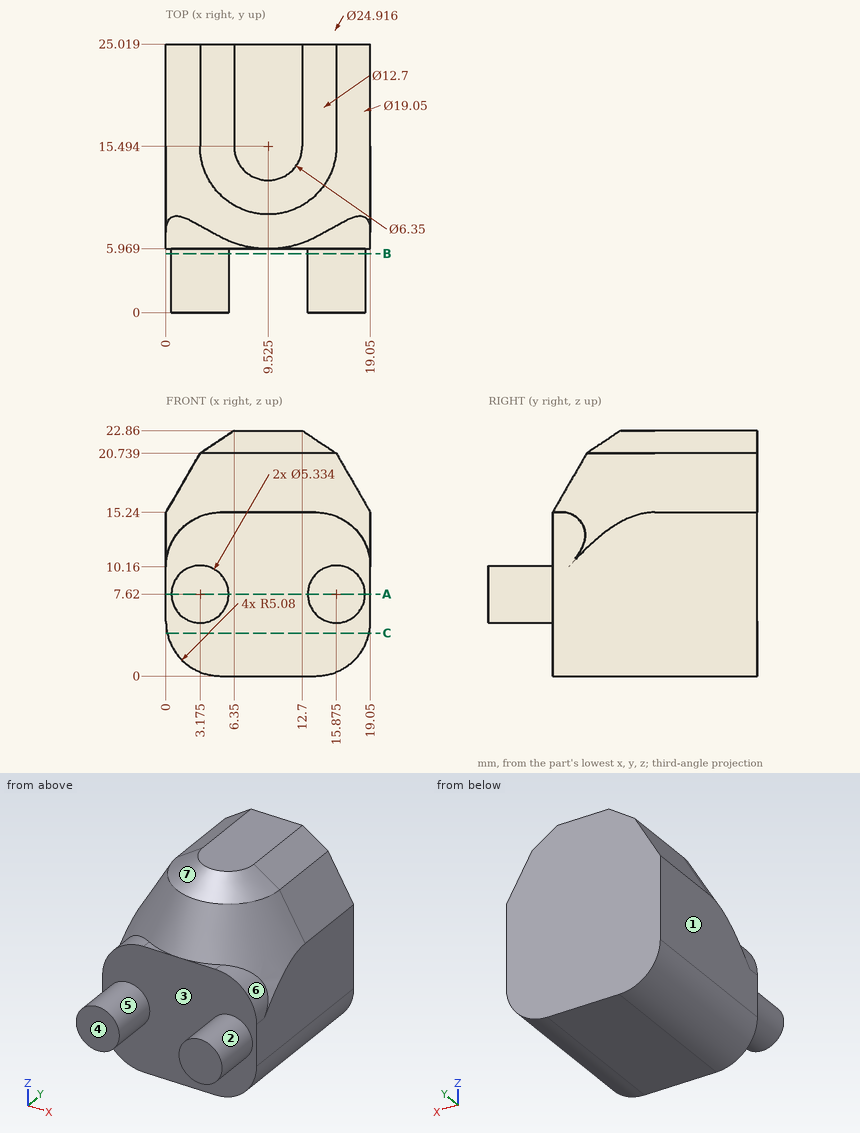
Drawing for the job (mm, zero at the part's lowest x, y, z). A direction names the side the tool comes from. Give positions to 0.01 mm unless a question says otherwise; leave off trailing zeros. Loops run counter-clockwise (first coordinate to the right, second up) from the corner with the lowest first, then second, coordinate; pieces in that order, holes last.
(1) Drill centre lines: line 1 along Y through (x, z) = (12.5, 10.5); line 2 along X through (y, z) = (2.5, 6.75); line 3 along Z through (x, y) = (3, 4.75). Where is each one in solid material? Low to high.
Return value:
line 1: y = 5.97 to 25.02
line 2: x = 0.65 to 5.7, 13.35 to 18.4
line 3: z = 4.96 to 10.28
(2) Pin check, flat tips, straight feed: pin 1 (5 mm diameter, centred on x = 6, y = 20, fed in from +Z); pin 2 (0.6 mm diameter, centred on x = 8, y = 6.5, fed in from +Z); pin 3 (2 mm diameter, centred on y = 11.5, z = 3, fed in from +X); pin 4 (0.9 mm diameter, centred on x = 12, y = 6.5, fed in from +Z). Stop position of each tip, or through.
Return value:
pin 1: stops at z = 22.86
pin 2: stops at z = 16.46
pin 3: stops at x = 18.93
pin 4: stops at z = 16.36
(3) Pull direction X, two halves, no side cores. Call the marked faces 1, 2, 3 and 4: pulls with the +X half, pulls with the -X half, needs draft (parallel to the pull), parting line crosses it, or undercut.
Return value:
face 1: pulls with the -X half
face 2: undercut
face 3: undercut
face 4: needs draft
(4) 3-axis set-ups, long thin cutter, end or side, ignore diameter. For the marked faces 5, 6 and 7: which of +Z, -Z, +X, -X, +Y, -Y reach the whole face in a straight line?
Return value:
face 5: -Y
face 6: +Z, +X, -Y
face 7: +Z, -Y
(5) Band-saw the part on A-A (z = 7.62). Write the cut outline in (x, y).
Return value:
outline: (0, 5.97) - (0.51, 5.97) - (0.51, 0) - (5.84, 0) - (5.84, 5.97) - (13.21, 5.97) - (13.21, 0) - (18.54, 0) - (18.54, 5.97) - (19.05, 5.97) - (19.05, 25.02) - (0, 25.02) - close
(6) Band-saw the part on C-C (z = 4). Write the cut outline in (x, y).
Return value:
outline: (0.12, 5.97) - (18.93, 5.97) - (18.93, 25.02) - (0.12, 25.02) - close
(7) Band-saw the part on B-B (y = 5.5). Write the cut outline in (x, z) (1 decimal).
Return value:
outline: circle Ø5.3 at (3.2, 7.6); circle Ø5.3 at (15.9, 7.6)
